Geometry: final body of the model. Coordinates: model frame, mm. Face numbers are marked on the shaded views. A direction names the side the tool comes from. Give positions to 0.01 mm unless a question says otherwise; leave off trailing zeros. Write each loop counter-clockwise with the first axis right and the second up, starting at its lowest first coordinate (ties: lowest second). Pieces come first, ordered by that corner, then holes. Notation, with made-up numbers: (76.25, 2.25) -> (106.25, 2.25) arc R27 ccw to (106.25, 37.25) -> close; hole circle Ø8 at (-14, 19). An arc over 180 degrees is marked (long way). Use CSV: the item, a comma, the result in double quotes. Start each with the question number.
1) Section A-A (x = 36.5). Output: boundary loops of the cut face in (y, z).
2) Contact query for flat-ended pins moving along their axis: P1, Ø12, axis at x = 25.5, z = 36.5, coming from the -Y side; P2, Ø11, axis at y = -23.5, z = -1, coming from the +X side; P3, Ø3, axis at x = 16.5, z = 6.5, coming from the +Y side; P4, Ø5.5, axis at x = -59.5, y = -15.5, coming from the +Z side. Output: stop coordinate, or through.
3) Section B-B (z = -4.5). Output: boundary loops of the cut face in (x, y), plus the area to 3 significant figures.
4) Section C-C (y = -9.5). Output: boundary loops of the cut face in (x, z) (1 decimal), plus the area to 3 significant figures.
5) Draft query along X for the marked faces 1, 2, 3 and 4. Return one class per face: pulls with the +X half, pulls with the -X half, needs draft (parallel to the pull), parting line crosses it, or undercut.
6) Material intervals for line 1 (Y direction, x = -36.5, z = 6.5); line 2 (Z direction, x = -12.5, y = -17); line 3 (X direction, y = -14.5, z = 9), sorted ascending. Write a range as [from, to].
7) Section D-D (y = -20.5). Output: boundary loops of the cut face in (x, z), plus the area to 3 significant figures.
8) Set-up query: the marked faces 5, 6 and 7. Return all of +Z, -Z, +X, -X, +Y, -Y with unobstructed straight access to the full face (end or side cutting, diameter ignored); none if empty.
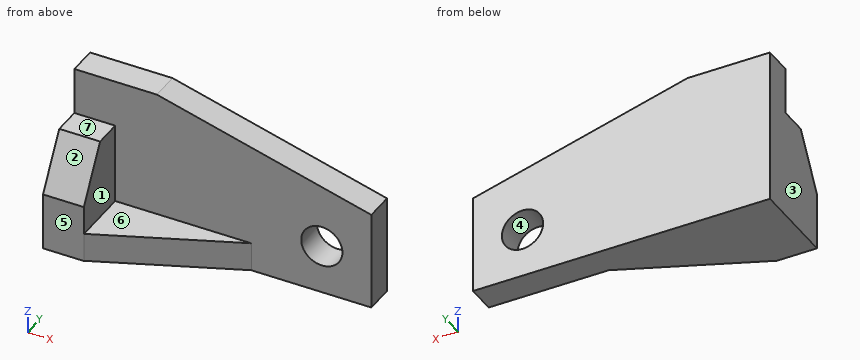
```python
from build123d import *

# Parameters (mm, degrees)
F0_R     = 7.9375
F0_W     = 15.7160045163
F0_H     = 42.1948071688
F1_DEPTH = 11.1125
F2_DEPTH = 33.3375
F4_DEPTH = 25.4
F5_W     = 52.3748
F5_H     = 11.1125
F6_DEPTH = 22.098
F8_DEPTH = 25.4


with BuildPart() as f1:
    # F0 (on Front) → F1 (new body)
    with BuildSketch(Plane.XZ):
        Polygon((-31.6839508394, 46.4698135108), (-63.4320186035, 46.4698135108), (-63.4320186035, 28.3396206796), (-47.7160140872, 28.3396206796), (-47.7160140872, -13.8551864892), (50.8660491606, -13.8551864892), (50.8660491606, 24.3506076756), align=None)
        with Locations((31.8160491606, 5.1003992379)):
            Circle(F0_R, mode=Mode.SUBTRACT)
        with Locations((-55.5740163454, 7.2422170952)):
            Rectangle(F0_W, F0_H)
    extrude(amount=F1_DEPTH)

    # F0 (on Front) → F2 (join)
    with BuildSketch(Plane.XZ):
        with Locations((-55.5740163454, 7.2422170952)):
            Rectangle(F0_W, F0_H)
    extrude(amount=F2_DEPTH)

    # F3 (on face) → F4 (cut)
    with BuildSketch(Plane.YZ.offset(-47.7160140872)):
        Polygon((-33.3375, 28.3396206796), (-33.3375, 8.3698135108), (-21.8079264554, 28.3396206796), align=None)
    extrude(amount=-F4_DEPTH, mode=Mode.SUBTRACT)

    # F5 (on face) → F6 (join)
    with BuildSketch(Plane.XZ.offset(11.1125)):
        with Locations((-21.5286140872, -8.2989364892)):
            Rectangle(F5_W, F5_H)
    extrude(amount=F6_DEPTH)

    # F7 (on face) → F8 (cut)
    with BuildSketch(Plane.XY.offset(-2.7426864892)):
        Polygon((4.6587859128, -11.1125), (-47.7160140872, -33.2105), (4.6587859128, -33.2105), align=None)
    extrude(amount=-F8_DEPTH, mode=Mode.SUBTRACT)


solid = f1.part
```
Answers follow:
1,outline,"(-11.11, -13.86) -> (0, -13.86) -> (0, -1.31) -> (-11.11, -1.31) -> close; (-11.11, 11.51) -> (0, 11.51) -> (0, 28.2) -> (-11.11, 28.2) -> close"
2,P1,"stops at y = -11.11"
2,P2,"stops at x = -12.34"
2,P3,"stops at y = 0"
2,P4,"stops at z = 28.34"
3,outline,"(-63.43, -33.34) -> (-47.72, -33.34) -> (-47.72, -33.21) -> (4.66, -11.11) -> (50.87, -11.11) -> (50.87, 0) -> (-63.43, 0) -> close"
3,area,"2,200 mm^2"
4,outline,"(-63.4, -13.9) -> (50.9, -13.9) -> (50.9, 24.4) -> (-31.7, 46.5) -> (-63.4, 46.5) -> close; hole circle Ø15.9 at (31.8, 5.1)"
4,area,"5,780 mm^2"
5,face 1,"pulls with the +X half"
5,face 2,"needs draft"
5,face 3,"pulls with the -X half"
5,face 4,"undercut"
6,line 1,"y = [-11.11, 0]"
6,line 2,"z = [-13.86, -2.74]"
6,line 3,"x = [-63.43, -47.72]"
7,outline,"(-63.43, -13.86) -> (-17.59, -13.86) -> (-17.59, -2.74) -> (-47.72, -2.74) -> (-47.72, 28.34) -> (-63.43, 28.34) -> close"
7,area,"998 mm^2"
8,face 5,"+Z, -Z, +X, -X, -Y"
8,face 6,"+Z, +X, -Y"
8,face 7,"+Z, +X, -X, -Y"
